Design review of the part built by this model. Coordinates are the model's own, in mm. Face numbers are marked on the shaded views. A direction names the side the tool comes from. Coordinates: 2 decimals unless noted, no trailing zeros. Order: outer loops, then holes, each group sorted by start corner. A loop starts at its lowest first (then second) coordinate and runs counter-clockwise, first axis right, second up. Notation, with made-up numbers: (18.25, -18.75) -> (67.25, -18.75) arc R28 ccw to (67.25, 15.25) -> close; hole circle Ø7 at (60, 45). An arc over 180 degrees is marked (long way). Use a Markdown table: item, result. Add a question column.
Q1. Wall thickness on probe 1 along X at (y, z) = (-305.5, -76); probe 2 along Y at (x, z) = (-111.5, -10); probe 3 along X at (y, z) = (-139, 99.5): over which ranges is each line inside the solid? List them lowest first.
Q2. Machinability: for the marked faces 1, 2 and 3, which of the approach directions +Z, -Z, +X, -X, +Y, -Y give a long, thin tool a straight path to every point of the face, cutting with its end or side? Answer none if there is none.
Q3. Add section B-B (x = 223). State the section outline as (y, z) points.
Q4. Insertion check: pin 1 (1.5 mm diameter, centred on y = -512.5, z = 3, fed in from +X); pin 2 (3 mm diameter, centred on y = -367.5, z = 1, fed in from -X); pin 3 (6 mm diameter, centred on x = 152.5, z = 122, fed in from -Y). Each pin has a flat end and moves straight along its axis. Give the tip position at first contact, or say it passes through.
Q5. Add section D-D (y = -564.5). State the section outline as (x, z) points.
Q6. Add section C-C (z = -41). State the section outline as (x, y) points, then the cut area to 3 significant figures.
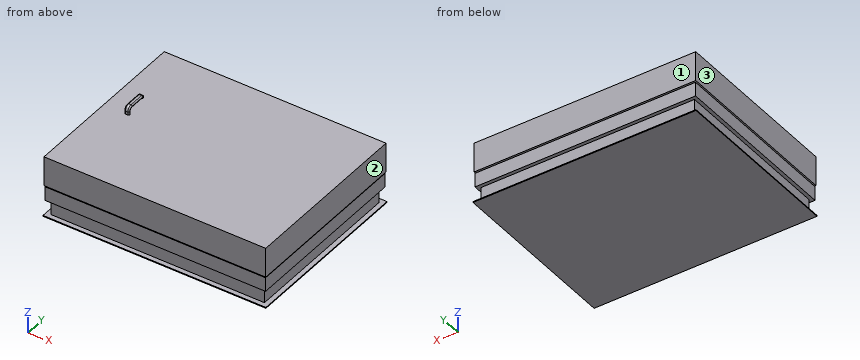
from build123d import *

# Parameters (mm, degrees)
F1_DEPTH = 754
F3_DEPTH = 999
F6_W     = 20
F6_H     = 10
F8_R     = 4.99999
F9_R     = 3


# Not quite as in the source:
# - a fillet or chamfer is up to 0.001 mm smaller than in the source, because OpenCascade refuses the exact size


with BuildPart() as f1:
    # F0 (on Front) → F1 (new body)
    with BuildSketch(Plane.XZ):
        Polygon((-477, -127), (-477, -131), (477, -131), (477, -127), (457, -127), (457, -61.5), (472, -61.5), (472, -1.5), (422, -1.5), (422, 4), (474.5, 4), (474.5, 131), (-474.5, 131), (-474.5, 4), (-422, 4), (-422, -1.5), (-472, -1.5), (-472, -61.5), (-457, -61.5), (-457, -127), align=None)
    extrude(amount=F1_DEPTH)

    # F2 (on face) → F3 (cut)
    with BuildSketch(Plane(origin=(-474.5, 0, 0), x_dir=(0, -1, 0), z_dir=(-1, 0, 0))):
        Polygon((754, -127), (754, -131), (765.5175328255, -131), (774.4438648224, 131), (751.5, 131), (751.5, 4), (699, 4), (699, -1.5), (749, -1.5), (749, -61.5), (734, -61.5), (734, -127), align=None)
        Polygon((55, 4), (2.5, 4), (2.5, 131), (-20.4438648224, 131), (-11.5175328255, -131), (0, -131), (0, -127), (20, -127), (20, -61.5), (5, -61.5), (5, -1.5), (55, -1.5), align=None)
    extrude(amount=-F3_DEPTH, mode=Mode.SUBTRACT)

    # F7: sweep along a path in F5
    with BuildLine(Plane(origin=(-374.5, 0, 0), x_dir=(0, -1, 0), z_dir=(-1, 0, 0))) as f7_path:
        Line((377, 131), (377, 144.4709453487))
        ThreePointArc((377, 144.4709453487), (372.6066017178, 155.0775470665), (362, 159.4709453487))
        Line((362, 159.4709453487), (297, 159.4709453487))
        ThreePointArc((297, 159.4709453487), (293.4644660941, 158.0064792547), (292, 154.4709453487))
        Line((292, 154.4709453487), (292, 150.8713660145))
    # F6 (on face) → F7 (sweep)
    with BuildSketch(Plane.XY.offset(131)):
        with Locations((-374.5, -377)):
            Rectangle(F6_W, F6_H)
    sweep(path=f7_path.line)

    # F8 (radius 5 in the source; OpenCascade refuses exactly that, so slightly less here)
    f8_edges = [f1.edges().sort_by_distance(p)[0] for p in [
        (-384.5, -329.5, 164.470945),
        (-384.5, -329.5, 154.470945),
        (-364.5, -329.5, 164.470945),
        (-364.5, -329.5, 154.470945),
    ]]
    fillet(f8_edges, radius=F8_R)

    # F9
    f9_edges = [f1.edges().sort_by_distance(p)[0] for p in [
        (-374.5, -287, 150.871366),
        (-374.5, -297, 150.871366),
        (-384.5, -294.499995, 150.871366),
    ]]
    fillet(f9_edges, radius=F9_R)


solid = f1.part
Established:
| question | item | result |
|---|---|---|
| 1 | probe 1 | -457 to 457 |
| 1 | probe 2 | -749 to -5 |
| 1 | probe 3 | -474.5 to 474.5 |
| 2 | face 1 | +Z, +X, -X, +Y |
| 2 | face 2 | +Z, +X, +Y, -Y |
| 2 | face 3 | +Z, -X, +Y, -Y |
| 3 | outline | (-754, -131) -> (0, -131) -> (0, -127) -> (-20, -127) -> (-20, -61.5) -> (-5, -61.5) -> (-5, -1.5) -> (-55, -1.5) -> (-55, 4) -> (-2.5, 4) -> (-2.5, 131) -> (-751.5, 131) -> (-751.5, 4) -> (-699, 4) -> (-699, -1.5) -> (-749, -1.5) -> (-749, -61.5) -> (-734, -61.5) -> (-734, -127) -> (-754, -127) -> close |
| 4 | pin 1 | x = 422 |
| 4 | pin 2 | x = -422 |
| 4 | pin 3 | y = -751.5 |
| 5 | outline | (-477, -131) -> (477, -131) -> (477, -127) -> (457, -127) -> (457, -61.5) -> (472, -61.5) -> (472, -1.5) -> (422, -1.5) -> (422, 4) -> (474.5, 4) -> (474.5, 131) -> (-474.5, 131) -> (-474.5, 4) -> (-422, 4) -> (-422, -1.5) -> (-472, -1.5) -> (-472, -61.5) -> (-457, -61.5) -> (-457, -127) -> (-477, -127) -> close |
| 6 | outline | (-472, -749) -> (472, -749) -> (472, -5) -> (-472, -5) -> close |
| 6 | area | 702,000 mm^2 |
